```python
from build123d import *

# Parameters (mm, degrees)
SKETCH1_R           = 22.225
BOSS_EXTRUDE1_DEPTH = 482.6
SKETCH2_R           = 25.4
BOSS_EXTRUDE2_DEPTH = 12.7
BOSS_EXTRUDE3_DEPTH = 76.2


with BuildPart() as part:
    # Sketch1 → Boss-Extrude1 (new body)
    with BuildSketch(Plane(origin=(0, 0, 0), x_dir=(1, 0, 0), z_dir=(0, 1, 0))):
        Circle(SKETCH1_R)
    extrude(amount=BOSS_EXTRUDE1_DEPTH)

    # Sketch2 → Boss-Extrude2 (add)
    with BuildSketch(Plane(origin=(0, 482.6, 0), x_dir=(1, 0, 0), z_dir=(0, 1, 0))):
        Circle(SKETCH2_R)
    extrude(amount=BOSS_EXTRUDE2_DEPTH)

    # Sketch3 → Boss-Extrude3 (add)
    with BuildSketch(Plane.XZ):
        with BuildLine():
            Line((-31.75, 0), (-31.75, -31.75))
            Line((-31.75, -31.75), (31.75, -31.75))
            Line((31.75, -31.75), (31.75, 0))
            ThreePointArc((31.75, 0), (0, 31.75), (-31.75, 0))
        make_face()
    extrude(amount=BOSS_EXTRUDE3_DEPTH)


solid = part.part
```
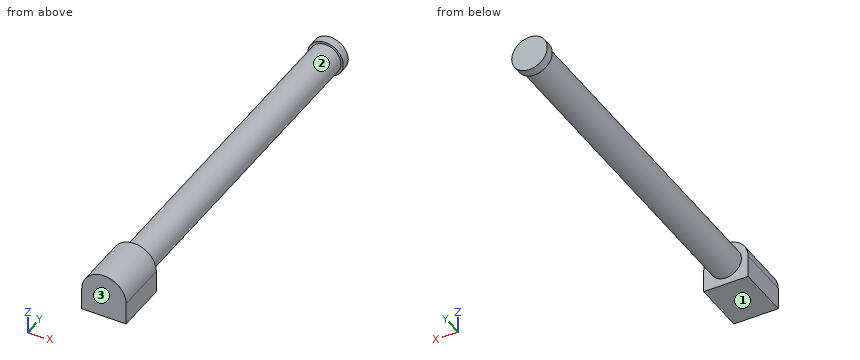
The listing builds one solid part. Answer for the finished solid, in the listing's coordinates (mm). Face numbers are marked on the shaded views. Round coordinates to 2 decimals unless told otherwise and drop trailing zeros. Loops run counter-clockwise (first coordinate to the right, second up) from the corner with the lowest first, then second, coordinate; pieces in that order, holes last.
1) Consider line 1 (Y direction, x = 17.5, z = -15); line 2 (Z direction, x = 0, y = 197.5) (3 decimals); line 3 (Y direction, x = 23.5, z = -14). Determine where each line is inside the solid, lowest interval first.
Outcome:
line 1: y = -76.2 to 0, 482.6 to 495.3
line 2: z = -22.225 to 22.225
line 3: y = -76.2 to 0
2) A cutting plane is placed at C-C on z = -16. Determine the outline of the cut face in (x, y).
Outcome:
outline: (-31.75, -76.2) - (31.75, -76.2) - (31.75, 0) - (15.43, 0) - (15.43, 482.6) - (19.73, 482.6) - (19.73, 495.3) - (-19.73, 495.3) - (-19.73, 482.6) - (-15.43, 482.6) - (-15.43, 0) - (-31.75, 0) - close
3) For a pull along Y with two mould halves and no side action, classify the marked faces 1, 2 and 3 as released by +Y, released by -Y, zero draft, split by the parting line, or undercut.
Outcome:
face 1: zero draft
face 2: undercut
face 3: released by -Y
4) Given P1, Ø6, axis at y = 230.5, z = -3, coming from the +X side (3 decimals); P2, Ø5, axis at y = 147, z = 19, coming from the -X side; P3, Ø2, axis at x = -1, y = 183, coming from the -Z side (3 decimals), each flat-ended and moving along its own axis, determine where each tip first touches the part or whether it passes through.
Outcome:
P1: stops at x = 22.225
P2: stops at x = -14.89
P3: stops at z = -22.225
5) A cutting plane is placed at B-B on y = 105.5. Determine the outline of the cut face in (x, z) (3 decimals), plus the area to 3 significant figures.
Outcome:
outline: circle Ø44.45 at (0, 0)
area: 1,550 mm2
6) A cutting plane is placed at A-A on x = 0. Determine the outline of the cut face in (y, z) (3 decimals), plus the area to 3 significant figures.
Outcome:
outline: (-76.2, -31.75) - (0, -31.75) - (0, -22.225) - (482.6, -22.225) - (482.6, -25.4) - (495.3, -25.4) - (495.3, 25.4) - (482.6, 25.4) - (482.6, 22.225) - (0, 22.225) - (0, 31.75) - (-76.2, 31.75) - close
area: 26,900 mm2
